```python
from build123d import *

# Parameters (mm, degrees)
F0_W     = 49.3294708431
F0_H     = 25.266315788
F1_DEPTH = 7.62
F2_SIZE2 = 7.61999
F2_SIZE  = 2.53999


# Not quite as in the source:
# - a fillet or chamfer is up to 0.001 mm smaller than in the source, because OpenCascade refuses the exact size


with BuildPart() as f1:
    # F0 (on Front) → F1 (new body)
    with BuildSketch(Plane.XZ):
        Rectangle(F0_W, F0_H)
    extrude(amount=F1_DEPTH)

    # F2 (size 2.54 and 7.62 in the source; OpenCascade refuses exactly that, so slightly less here)
    f2_edges = [f1.edges().sort_by_distance(p)[0] for p in [
        (0, -7.62, 12.633158),
        (24.664735, -7.62, 0),
        (-24.664735, -7.62, 0),
        (0, -7.62, -12.633158),
    ]]
    f2_side = f1.faces().sort_by_distance((0, -7.62, 0))[0]
    chamfer(f2_edges, length=F2_SIZE, length2=F2_SIZE2, reference=f2_side)


solid = f1.part
```
Build history of the part. All positions in model axes, mm. Give positions to 0.01 mm unless a question says otherwise; leave off trailing zeros. Order: outer loops, then holes, each group sorted by start corner. A loop starts at its lowest first (then second) coordinate and runs counter-clockwise, first axis right, second up. Notation, with made-up numbers: M -29.75,26 L 28.25,26 A4 ccw 28.25,33 Z; hole C 23.5,-31.5 d4. An arc over 180 degrees is marked long. Return JSON: item names as keys, results as strings.
Q1. Band-saw the part on C-C (y = -4.25). Give the cut face in (x, z), then the cut area to 3 significant figures.
Answer list:
{"outline": "M -23.25,-11.22 L 23.25,-11.22 L 23.25,11.22 L -23.25,11.22 Z", "area": "1,040 mm^2"}
Q2. Wall check: probe 1 along X at (y, z) = (-1.5, 4.75); probe 2 along Z at (x, y) = (-9.5, -6); probe 3 along X at (y, z) = (-5.25, 1.25). Give the ranges that are in metal, low to high. Write a range as from..to.
Answer list:
{"probe 1": "x = -24.16..24.16", "probe 2": "z = -10.63..10.63", "probe 3": "x = -22.91..22.91"}
Q3. Band-saw the part on D-D (y = -1). Give the cut face in (x, z), then the cut area to 3 significant figures.
Answer list:
{"outline": "M -24.33,-12.3 L 24.33,-12.3 L 24.33,12.3 L -24.33,12.3 Z", "area": "1,200 mm^2"}
Q4. Flat gauge pins, fed straight in: pin 1 (1.5 mm diameter, centred on x = -2.5, z = -7, fed in from +Y); pin 2 (1.5 mm diameter, centred on x = -5.5, y = -1, fed in from +Z); pin 3 (3 mm diameter, centred on x = -2.5, y = -4.5, fed in from +Z). Where does each tip first touch, or does it go through?
Answer list:
{"pin 1": "stops at y = 0", "pin 2": "stops at z = 12.55", "pin 3": "stops at z = 11.63"}
